from build123d import *

# Parameters (mm, degrees)
SKETCH1_R           = 1.25
BOSS_EXTRUDE1_DEPTH = 9
SKETCH2_R           = 2.5
BOSS_EXTRUDE2_DEPTH = 2
CUT_EXTRUDE1_DEPTH  = 1
FILLET1_R           = 0.5


with BuildPart() as part:
    # Sketch1 → Boss-Extrude1 (new body)
    with BuildSketch(Plane.XY):
        Circle(SKETCH1_R)
    extrude(amount=-BOSS_EXTRUDE1_DEPTH)

    # Sketch2 → Boss-Extrude2 (add)
    with BuildSketch(Plane.XY):
        Circle(SKETCH2_R)
    extrude(amount=BOSS_EXTRUDE2_DEPTH)

    # Sketch3 → Cut-Extrude1 (cut)
    with BuildSketch(Plane.XY.offset(2)):
        Polygon((1.283002505, 0), (0.641501252, 1.111112762), (-0.641501252, 1.111112762), (-1.283002505, 0), (-0.641501252, -1.111112762), (0.641501252, -1.111112762), align=None)
    extrude(amount=-CUT_EXTRUDE1_DEPTH, mode=Mode.SUBTRACT)

    # Fillet1
    fillet1_edges = [part.edges().sort_by_distance(p)[0] for p in [
        (-2.5, 0, 0),
        (-2.5, 0, 2),
    ]]
    fillet(fillet1_edges, radius=FILLET1_R)


solid = part.part
Verification items for the finished model (mm, model axes). A direction names the side the tool comes from. Coordinates: 2 decimals unless noted, no trailing zeros. Order: outer loops, then holes, each group sorted by start corner. A loop starts at its lowest first (then second) coordinate and runs counter-clockwise, first axis right, second up. Notation, with made-up numbers: M 19,4.25 L 71,4.25 A11 cw 71,25.25 Z; hole C 48,-7 d5. An arc over 180 degrees is marked long. One line per item, written item: value. Start each with the question number.
Item 1: Gauge pin test, flat ends, axial feed: pin 1 (0.5 mm diameter, centred on x = -0.5, z = 1.5, fed in from -Y); pin 2 (1.5 mm diameter, centred on y = -1.5, z = -2, fed in from +X); pin 3 (0.7 mm diameter, centred on x = 0.5, y = 0.5, fed in from +Z). Record the tip position at first contact, or that the pin passes through.
Item 2: Sectioned sample at A-A (x = 0). Enter the section's corners in (y, z).
Item 3: Scan lines: probe 1 along Z at (x, y) = (-0.4, 0.75); probe 2 along Z at (x, y) = (0.15, -2.05); probe 3 along X at (y, z) = (0.75, 1.5). Record each from-to range of solid material in increasing order.
Item 4: Access from +Z, -Z, +X, -X, +Y, -Y to the whole of each face (thin tool, end or side, straight path). Record for faces 1 (the flat face through (1, 1, 0)), 2 (the flat face through (1, -1, 2)), 3 (the flat face through (0, 1.111, 1.5)).
Item 5: Mould release check, pull along X, two halves, no side actions. Record for faces 4 (the flat face through (0, 0, -9)), 5 (the flat face through (0.967, 0.548, 1.507)), 6 (the cylindrical face through (-0.54, -2.44, 0.99)): released by +X, released by -X, zero draft, split by the parting line, or undercut.
Item 6: Sectioned sample at B-B (z = -5.5). Enter the section's corners in (x, y).
Conclusion:
1. pin 1: stops at y = -2.49
1. pin 2: stops at x = 1
1. pin 3: stops at z = 1
2. outline: M -2.5,0.5 A0.5 ccw -2,0 L -1.25,0 L -1.25,-9 L 1.25,-9 L 1.25,0 L 2,0 A0.5 ccw 2.5,0.5 L 2.5,1.5 A0.5 ccw 2,2 L 1.11,2 L 1.11,1 L -1.11,1 L -1.11,2 L -2,2 A0.5 ccw -2.5,1.5 Z
3. probe 1: z = -9 to 1
3. probe 2: z = 0 to 2
3. probe 3: x = -2.38 to -0.85, 0.85 to 2.38
4. face 1: -Z
4. face 2: +Z, +X, -X, +Y, -Y
4. face 3: +Z
5. face 4: zero draft
5. face 5: undercut
5. face 6: split by the parting line
6. outline: C 0,0 d2.5
